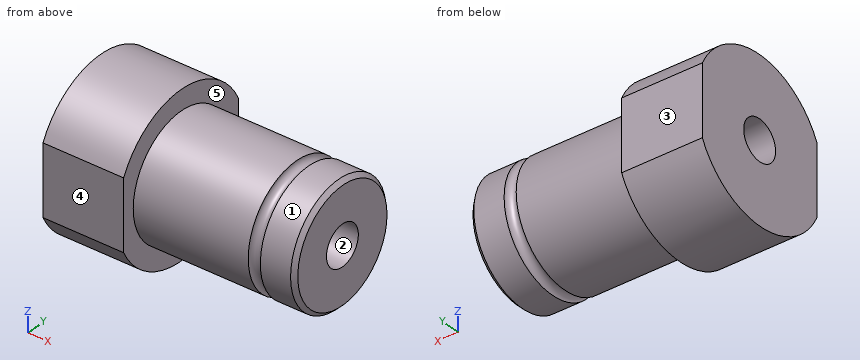
from build123d import *

# Parameters (mm, degrees)
F2_SIZE  = 1
F4_DEPTH = 60.001
F5_R     = 5
F6_DEPTH = 60.001
F7_R     = 1.5


with BuildPart() as f1:
    # F0 (on Top) → F1 (revolve)
    with BuildSketch(Plane.XY):
        Polygon((0, 20), (0, 0), (60, 0), (60, 15), (20, 15), (20, 20), align=None)
    revolve(axis=Axis((30, 0, 0), (-1, 0, 0)))

    # F2
    f2_edges = [f1.edges().sort_by_distance(p)[0] for p in [
        (60, -15, 0),
    ]]
    chamfer(f2_edges, length=F2_SIZE)

    # F3 (on face) → F4 (cut, through all)
    with BuildSketch(Plane(origin=(0, 0, 0), x_dir=(0, -1, 0), z_dir=(-1, 0, 0))):
        with BuildLine():
            Line((-18, -8.7177978871), (-18, 8.7177978871))
            ThreePointArc((-18, 8.7177978871), (-20, 0), (-18, -8.7177978871))
        make_face()
        with BuildLine():
            ThreePointArc((20, 0), (19.4935886896, 4.472135955), (18, 8.7177978871))
            Line((18, 8.7177978871), (18, -8.7177978871))
            ThreePointArc((18, -8.7177978871), (19.4935886896, -4.472135955), (20, 0))
        make_face()
    extrude(amount=-F4_DEPTH, mode=Mode.SUBTRACT)

    # F5 (on face) → F6 (cut, through all)
    with BuildSketch(Plane(origin=(0, 0, 0), x_dir=(0, -1, 0), z_dir=(-1, 0, 0))):
        Circle(F5_R)
    extrude(amount=-F6_DEPTH, mode=Mode.SUBTRACT)

    # F7 (on Front) → F8 (revolve, cut)
    with BuildSketch(Plane.XZ):
        with Locations((50, 15)):
            Circle(F7_R)
    revolve(axis=Axis((60, 0, 0), (-1, 0, 0)), mode=Mode.SUBTRACT)


solid = f1.part
Design review of the part built by this model. Coordinates are the model's own, in mm. Face numbers are marked on the shaded views. A direction names the side the tool comes from. Give positions to 0.01 mm unless a question says otherwise; leave off trailing zeros. Write each loop counter-clockwise with the first axis right and the second up, starting at its lowest first coordinate (ties: lowest second). Pieces come first, ordered by that corner, then holes. Notation, with made-up numbers: M 40,87.5 L 93,87.5 A19 ccw 93,96.5 Z; hole C -29.5,10 d10. An arc over 180 degrees is marked long. Answer as a JSON object with one key per item and string values. Group by question number.
1) Mouldability with a two-part tool opening along Y and no side actions: class the marked faces 1, 2 and 3 as released by +Y, released by -Y, zero draft, split by the parting line, or undercut.
2) Clearance check with flat-ended pins moving along their axes: pin 1 Ø12 at (x, y) = (38.5, 2) entering from -Z; pin 2 Ø10 at (x, y) = (35, 10.5) entering from -Z; pin 3 Ø1.5 at (x, z) = (31.5, -10) entering from -Y. State where each tip first meets the part, or that it passes through.
3) We need section C-C (x = 33). Give the boundary of the cut face in (y, z), and give its area (3 significant figures).
4) We need section B-B (y = 0). Give the boundary of the cut face in (x, z).
5) Tool access review of the marked faces 4 and 5: name each direction out of +Z, -Z, +X, -X, +Y, -Y from which nothing blocks a thin tool from reaching the whole face with its end or side.
6) For line 1 along Z through (x, y) = (23, 0); line 2 along X through (y, z) = (-12, 11.5); line 3 along Z through (x, y) = (30, 3.5), list the stretches that pass through material, from the lowest coordinate up.
7) We need section A-A (z = 0). Give the boundary of the cut face in (x, y), and give its area (3 significant figures).
Answer key:
{
 "1": {"face 1": "split by the parting line", "face 2": "undercut", "face 3": "released by +Y"},
 "2": {"pin 1": "stops at z = -15", "pin 2": "stops at z = -13.96", "pin 3": "stops at y = -11.81"},
 "3": {"outline": "C 0,0 d30; hole C 0,0 d10", "area": "628 mm²"},
 "4": {"outline": "M 0,-20 L 20,-20 L 20,-15 L 48.5,-15 A1.5 cw 51.5,-15 L 59,-15 L 60,-14 L 60,-5 L 0,-5 Z; M 0,5 L 60,5 L 60,14 L 59,15 L 51.5,15 A1.5 cw 48.5,15 L 20,15 L 20,20 L 0,20 Z"},
 "5": {"face 4": "+Z, -Z, +X, -X, -Y", "face 5": "+X"},
 "6": {"line 1": "z = -15 to -5, 5 to 15", "line 2": "x = 0 to 20", "line 3": "z = -14.59 to -3.57, 3.57 to 14.59"},
 "7": {"outline": "M 0,-18 L 20,-18 L 20,-15 L 48.5,-15 A1.5 cw 51.5,-15 L 59,-15 L 60,-14 L 60,-5 L 0,-5 Z; M 0,5 L 60,5 L 60,14 L 59,15 L 51.5,15 A1.5 cw 48.5,15 L 20,15 L 20,18 L 0,18 Z", "area": "1,310 mm²"}
}
